Build history of the part. All positions in model axes, mm. Face numbers are marked on the shaded views. Round coordinates to 2 decimals unless told otherwise and drop trailing zeros. Write each loop counter-clockwise with the first axis right and the second up, starting at its lowest first coordinate (ties: lowest second). Pieces come first, ordered by that corner, then holes. Notation, with made-up numbers: (18.5, 65) -> (38.5, 65) arc R13 ccw to (38.5, 74) -> close; hole circle Ø6 at (-12.75, 21). An arc over 180 degrees is marked (long way). Return JSON: item names as keys, results as strings.
from build123d import *

# Parameters (mm, degrees)
F0_R      = 28.45
F1_DEPTH  = 230
F2_R      = 25.5
F3_DEPTH  = 90
F8_R      = 8
F9_DEPTH  = 5
F11_R     = 25
F11_R_2   = 15
F12_DEPTH = 12.5


with BuildPart() as f1:
    # F0 (on Front) → F1 (new body)
    with BuildSketch(Plane.XZ):
        Circle(F0_R)
    extrude(amount=F1_DEPTH)

    # F2 (on face) → F3 (join)
    with BuildSketch(Plane.XZ.offset(230)):
        Circle(F2_R)
    extrude(amount=F3_DEPTH)

    # F4 (on Right) → F5 (revolve)
    with BuildSketch(Plane.YZ):
        Polygon((-285, -21.45), (-285, 0), (-320, 0), (-320, -25.5), align=None)
    revolve(axis=Axis((0, -302.5, 0), (0, 1, 0)))

    # F6 (on Right) → F7 (revolve)
    with BuildSketch(Plane.YZ):
        Polygon((8, 0), (0, 0), (0, -19.82), (8, -8), align=None)
    revolve(axis=Axis((0, 4, 0), (0, 1, 0)))

    # F8 (on face) → F9 (join)
    with BuildSketch(Plane(origin=(0, 8, 0), x_dir=(-1, 0, 0), z_dir=(0, 1, 0))):
        Circle(F8_R)
    extrude(amount=F9_DEPTH)

    # F11 (on Right) → F12 (join, symmetric)
    with BuildSketch(Plane.YZ):
        with Locations((-340, 0)):
            Circle(F11_R)
        with Locations((-340, 0)):
            Circle(F11_R_2, mode=Mode.SUBTRACT)
        with Locations((33, 0)):
            Circle(F11_R)
        with Locations((33, 0)):
            Circle(F11_R_2, mode=Mode.SUBTRACT)
    extrude(amount=F12_DEPTH, both=True)


solid = f1.part
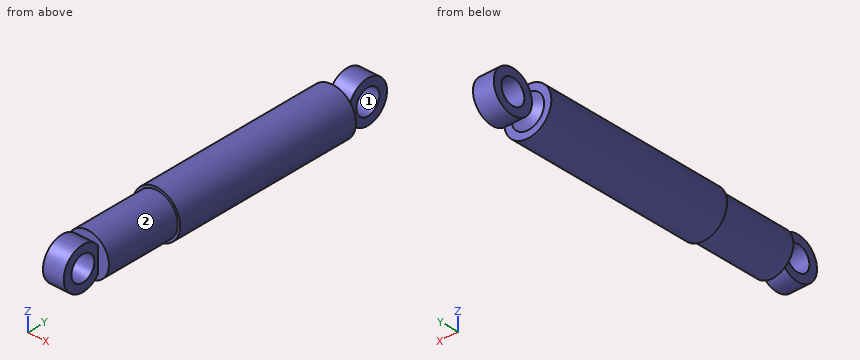
Q1. Saw through at B-B on x = 0. List the corners of the cut face in (y, z).
Verdict:
{"outline": "(-320, -25.5) -> (-230, -25.5) -> (-230, -28.45) -> (0, -28.45) -> (0, -19.82) -> (8, -8) -> (9.31, -8) arc R25 ccw (long way) to (9.31, 8) -> (8, 8) -> (0, 19.82) -> (0, 28.45) -> (-230, 28.45) -> (-230, 25.5) -> (-320, 25.5) -> (-320, 15) arc R25 ccw (long way) to (-320, -15) -> close; hole circle Ø30 at (-340, 0); hole circle Ø30 at (33, 0)"}
Q2. Two-plate mould, pull along Z, no slides. Class the marked faces 1 and 2: +Z half, -Z half, draft (parallel to the pull), parting line (faces both ways), or undercut.
Verdict:
{"face 1": "undercut", "face 2": "parting line"}
Q3. Pin check, flat tips, straight feed: pin 1 Ø5 at (y, z) = (-51.5, -0.5) entering from +X; pin 2 Ø6 at (x, y) = (9.5, -194.5) entering from +Z; pin 3 Ø4 at (x, y) = (-8, -18.5) entering from +Z; pin 4 Ø3 at (x, y) = (13.5, -203) entering from +Z. Stop position of each tip, or through.
Verdict:
{"pin 1": "stops at x = 28.45", "pin 2": "stops at z = 27.7", "pin 3": "stops at z = 27.81", "pin 4": "stops at z = 25.8"}
Q4. Saw through at C-C on y = -182.5. List the corners of the cut face in (x, z).
Verdict:
{"outline": "circle Ø56.9 at (0, 0)"}
Q5. Saw through at A-A on y = -340. List the corners of the cut face in (x, z).
Verdict:
{"outline": "(-12.5, -25) -> (12.5, -25) -> (12.5, -15) -> (-12.5, -15) -> close; (-12.5, 15) -> (12.5, 15) -> (12.5, 25) -> (-12.5, 25) -> close"}
Q6. Saw through at D-D on y = -260.5. List the corners of the cut face in (x, z), then the cut area to 3 significant figures.
Verdict:
{"outline": "circle Ø51 at (0, 0)", "area": "2,040 mm²"}
Q7. Wall check: L1, parallel to Z at x = 5, y = 33; L2, parallel to Y at x = -3, z = -18; L3, parallel to Y at x = -5.5, z = -22.5. Give the ranges that are in metal, low to high.
Verdict:
{"L1": "z = -25 to -15, 15 to 25", "L2": "y = -357.35 to -322.65, -320 to 1.06, 15.65 to 50.35", "L3": "y = -350.9 to -329.1, -320 to 0, 22.1 to 43.9"}
